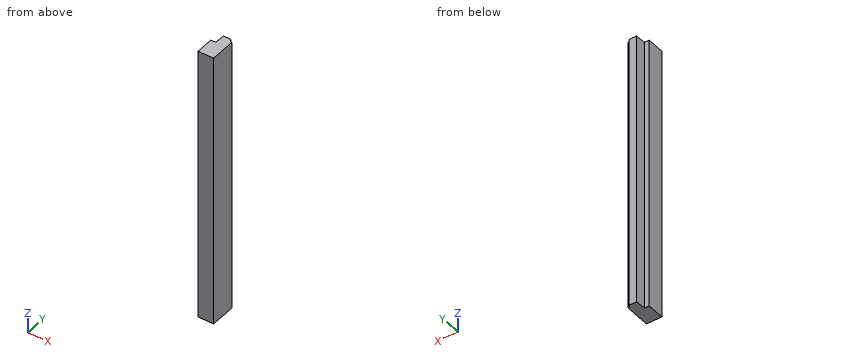
Autodesk Inventor part; units mm, degrees
ref_plane "YZ Plane" through (0, 0, 0) normal (1, 0, 0) x (0, 1, 0)
ref_plane "XZ Plane" through (0, 0, 0) normal (0, 1, 0) x (-1, 0, 0)
ref_plane "XY Plane" through (0, 0, 0) normal (0, 0, 1) x (1, 0, 0)
sketch "スケッチ1" plane through (43.5, 1.6, 26.25) normal (0, 0, -1) x (-1, 0, 0)
  line L0 (-3, 0.5001) -> (-3, -0.5)
  line L1 (0, -0.5) -> (0, 0.4999)
  line L2 (0, -0.0868) -> (0, 2.9)
  line L3 (-3, -0.0868) -> (-3, 4.4)
  circle A0 centre (-3, 4.9) radius 0.5
  line L4 (-1, 4.9) -> (-2.5, 4.9)
  line L5 (-1, 4.9) -> (-0.9302, 2.9)
  line L6 (-0.9302, 2.9) -> (0, 2.9)
  line L7 (-3, -0.5) -> (0, -0.5)
  point P0 (43.5, -1.6)
  point P1 (-2.5, 4.9)
extrude "押し出し1" add sketch "スケッチ1" along normal blind 54 contours L3 A0 L4 L5 L6 L2 L1 L7 L0
properties part number "base_01"
Verification items for the finished model (mm, model axes). Round coordinates to 2 decimals unless told otherwise and drop trailing zeros. Loops run counter-clockwise (first coordinate to the right, second up) from the corner with the lowest first, then second, coordinate; pieces in that order, holes last. Notation, with made-up numbers: (54.5, -22) - (72.5, -22) arc R18 cw to (72.5, 1) - close; hole circle Ø1 at (12, 15.25). An arc over 180 degrees is marked (long way). Use one line per item in the form item = value.
1. Section check A-A on z = -10.5. Record the cut outline in (x, y), and give its area (3 significant figures).
A:
outline = (43.5, 1.1) - (46.5, 1.1) - (46.5, 6) arc R0.5 cw to (46, 6.5) - (44.5, 6.5) - (44.43, 4.5) - (43.5, 4.5) - close
area = 14.1 mm²
2. Section check B-B on y = 5.35. Record the cut outline in (x, z), and give its area (3 significant figures).
A:
outline = (44.46, -27.75) - (46.5, -27.75) - (46.5, 26.25) - (44.46, 26.25) - close
area = 110 mm²
3. Scan lines: probe 1 along Y at (x, z) = (44.35, -4); probe 2 along X at (y, z) = (5.2, -3.5); probe 3 along Y at (x, z) = (46.35, -19). Record each from-to range of solid material in increasing order.
A:
probe_1 = 1.1 to 4.5
probe_2 = 44.45 to 46.5
probe_3 = 1.1 to 6.02
